```python
from build123d import *

# Parameters (mm, degrees)
F0_W     = 75.254161
F0_H     = 23.219683
F1_DEPTH = 76.2
F2_R     = 12.016458
F3_DEPTH = 101.6
F4_R     = 68.933228
F5_DEPTH = 101.6
F6_R     = 25.4
F7_R     = 12.7


with BuildPart() as f1:
    # F0 (on Front) → F1 (new body)
    with BuildSketch(Plane.XZ):
        with Locations((0.559511, -43.362062)):
            Rectangle(F0_W, F0_H)
    extrude(amount=F1_DEPTH)

    # F2 (on face) → F3 (join)
    with BuildSketch(Plane.XY.offset(-31.752221)):
        with Locations((0, -40.984146)):
            Circle(F2_R)
    extrude(amount=F3_DEPTH)

    # F4 (on face) → F5 (join)
    with BuildSketch(Plane.XY.offset(69.847779)):
        with Locations((0, -40.984146)):
            Circle(F4_R)
    extrude(amount=F5_DEPTH)

    # F6
    f6_edges = [f1.edges().sort_by_distance(p)[0] for p in [
        (-68.933228, -40.984146, 171.447779),
        (-68.933228, -40.984146, 69.847779),
    ]]
    fillet(f6_edges, radius=F6_R)

    # F7
    f7_edges = [f1.edges().sort_by_distance(p)[0] for p in [
        (38.186591, -76.2, -43.362062),
        (38.186591, 0, -43.362062),
        (-37.06757, -76.2, -43.362062),
        (0.559511, -76.2, -54.971904),
        (38.186591, -38.1, -54.971904),
        (0.559511, 0, -54.971904),
        (-37.06757, -38.1, -54.971904),
        (-37.06757, 0, -43.362062),
    ]]
    fillet(f7_edges, radius=F7_R)


solid = f1.part
```
Here's how the part is built. I have some questions about the finished solid (model axes, mm). A direction names the side the tool comes from. Round coordinates to 2 decimals unless told otherwise and drop trailing zeros. Write each loop counter-clockwise with the first axis right and the second up, starting at its lowest first coordinate (ties: lowest second). Pieces come first, ordered by that corner, then holes.
Q1. Will these pins go through, and if not, where does the flat tip stop? P1, Ø3, axis at x = -5.5, z = -35, coming from the +Y side; P2, Ø5.5, axis at x = 13, z = -34.5, coming from the -Y side; P3, Ø6, axis at y = -38, z = 16, coming from the -X side.
Q2. Which directions (+Z, -Z, +X, -X, +Y, -Y) give clear straight access to the entire face, cutting with the end or side of a thin tool? Please do faces 1 (the flat face through (0, 0, -37)), 2 (the cylindrical face through (34.368, -3.622, -36.938)), 3 (the flat face through (-37.068, -38, -37)).
Q3. If we section it at A-A on x = 0: Write out the boundary of the cut face in (y, z).
Q4. Please list where these lines run through material, in increasing order: probe 1 along Z at (x, y) = (-23.5, -27); probe 2 along X at (y, z) = (-42, 43); probe 3 along Z at (x, y) = (14.5, -1).
Q5. If we section it at B-B on z = 11.5: Write out the boundary of the cut face in (x, y), plus the area to 3 significant figures.
Q6. If we mould it in two halves opening along Z, with no side actions, what happens to faces 4 (the flat face through (9, -50, 69.848)), 5 (the cylindrical face through (-2.605, -52.715, 18.337)), 6 (the flat face through (38.187, -38, -37)), 7 (the cylindrical face through (34.57, -38.46, -51.15))? For each: +Z half, -Z half, draft (parallel to the pull), parting line (faces both ways), or undercut.
Answer below:
1. P1: stops at y = 0
1. P2: stops at y = -76.2
1. P3: stops at x = -12.02
2. face 1: -Z, +X, -X, +Y
2. face 2: -Z, +X, +Y
2. face 3: -Z, -X, +Y, -Y
3. outline: (-109.92, 95.25) arc R25.4 ccw to (-84.52, 69.85) - (-53, 69.85) - (-53, -31.75) - (-76.2, -31.75) - (-76.2, -42.27) arc R12.7 ccw to (-63.5, -54.97) - (-12.7, -54.97) arc R12.7 ccw to (0, -42.27) - (0, -31.75) - (-28.97, -31.75) - (-28.97, 69.85) - (2.55, 69.85) arc R25.4 ccw to (27.95, 95.25) - (27.95, 146.05) arc R25.4 ccw to (2.55, 171.45) - (-84.52, 171.45) arc R25.4 ccw to (-109.92, 146.05) - close
4. probe 1: z = -54.97 to -31.75, 69.85 to 171.45
4. probe 2: x = -11.97 to 11.97
4. probe 3: z = -47.21 to -31.75, 69.85 to 171.45
5. outline: circle Ø24.03 at (0, -40.98)
5. area: 454 mm2
6. face 4: undercut
6. face 5: undercut
6. face 6: draft
6. face 7: -Z half
